```python
from build123d import *

# Parameters (mm, degrees)
FILLET1_R = 0.3


with BuildPart() as part:
    # Sketch1 → Revolve1 (revolve)
    with BuildSketch(Plane.XY, mode=Mode.PRIVATE) as revolve1_sk:
        with BuildLine():
            Line((0, 3.5), (0, 13))
            Line((0, 13), (1.682055053, 11.614110106))
            ThreePointArc((1.682055053, 11.614110106), (2, 11.5), (2.317944947, 11.614110106))
            Line((2.317944947, 11.614110106), (4, 13))
            Line((4, 13), (4, 4.1))
            Line((4, 4.1), (1.5, 4.1))
            Line((1.5, 4.1), (1.5, 3.5))
            Line((1.5, 3.5), (0, 3.5))
        make_face()
    revolve(revolve1_sk.sketch.rotate(Axis((0, 0, 0), (1, 0, 0)), 90), axis=Axis((0, 0, 0), (1, 0, 0)))

    # Fillet1
    fillet1_edges = [part.edges().sort_by_distance(p)[0] for p in [
        (0, 0, -13),
        (4, 0, -13),
    ]]
    fillet(fillet1_edges, radius=FILLET1_R)


solid = part.part
```
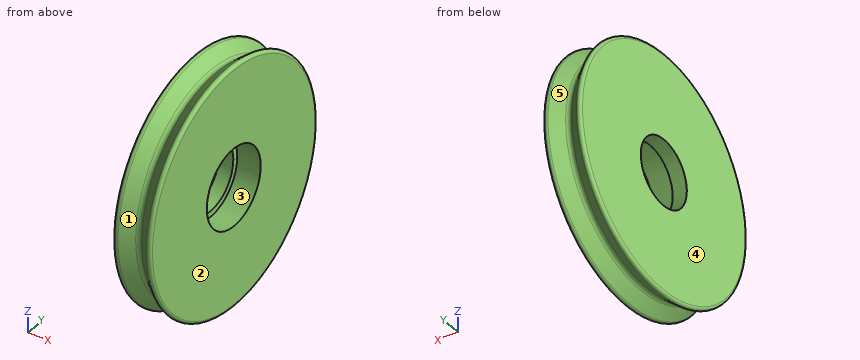
Could you check a few things on this model? Use its own coordinates, in mm. Face numbers are marked on the shaded views. A direction names the side the tool comes from. Give positions to 0.01 mm unless a question says otherwise; leave off trailing zeros. Order: outer loops, then holes, each group sorted by start corner. A loop starts at its lowest first (then second) coordinate and runs counter-clockwise, first axis right, second up.
Q1. Suppose I cut it at C-C, the plane x = 0.8. Write out the boundary of the cut face in (y, z).
Q2. Suppose I cut it at A-A, the plane y = 0. Write out the boundary of the cut face in (x, z), and give its area (3 significant figures).
Q3. I'm going to push flat-ended pins straight in: P1, Ø1.5, axis at x = 2, z = 7, coming from the +Y side; P2, Ø2, axis at x = 2.5, z = 6, coming from the +Y side. Where does each tip first touch, or does it pass through?
Q4. We'd pull the mould along Z, two halves only. Please class the marked faces 3, 4 and 5: +Z half, -Z half, draft (parallel to the pull), parting line (faces both ways), or undercut.
Q5. Suppose I cut it at D-D, the plane x = 3.05. Write out the boundary of the cut face in (y, z).
Q6. If I drill on line 1 along X through (y, z) = (-11, 5.5); line 2 along Z through (x, y) = (2.55, -2.25); line 3 along Y through (x, z) = (0.4, 0), over which ranges is the centre line in solid material (lowest first)?
Q7. For the marked faces 1 and 2, which set-ups out of +Z, -Z, +X, -X, +Y, -Y let a thin tool reach every point of the face, with its end or its side?
Solution:
1. outline: circle Ø24.68 at (0, 0); hole circle Ø7 at (0, 0)
2. outline: (0, -12.36) arc R0.3 ccw to (0.49, -12.6) - (1.68, -11.61) arc R0.5 cw to (2.32, -11.61) - (3.51, -12.6) arc R0.3 ccw to (4, -12.36) - (4, -4.1) - (1.5, -4.1) - (1.5, -3.5) - (0, -3.5) - close; (0, 3.5) - (1.5, 3.5) - (1.5, 4.1) - (4, 4.1) - (4, 12.36) arc R0.3 ccw to (3.51, 12.6) - (2.32, 11.61) arc R0.5 cw to (1.68, 11.61) - (0.49, 12.6) arc R0.3 ccw to (0, 12.36) - close
2. area: 66.1 mm2
3. P1: stops at y = 9.87
3. P2: stops at y = 11.2
4. face 3: undercut
4. face 4: draft
4. face 5: parting line
5. outline: circle Ø24.43 at (0, 0); hole circle Ø8.2 at (0, 0)
6. line 1: x = 0 to 0.85, 3.15 to 4
6. line 2: z = -11.59 to -3.43, 3.43 to 11.59
6. line 3: y = -12.65 to -3.5, 3.5 to 12.65
7. face 1: none
7. face 2: +Z, -Z, +X, +Y, -Y
